Autodesk Inventor part; units mm, degrees
ref_plane "YZ Plane" through (0, 0, 0) normal (1, 0, 0) x (0, 1, 0)
ref_plane "XZ Plane" through (0, 0, 0) normal (0, 1, 0) x (-1, 0, 0)
ref_plane "XY Plane" through (0, 0, 0) normal (0, 0, 1) x (1, 0, 0)
sketch "Sketch1" plane through (0, 0, 0) normal (0, 1, 0) x (-1, 0, 0)
  line L0 (0, 0) -> (0, -2) construction
  line L1 (-2.5, 0) -> (-2.5, -2)
  line L2 (2.5, -2) -> (2.5, 0)
  arc A0 (2.5, 0) -> (-2.5, 0) centre (0, 0) ccw
  arc A1 (-2.5, -2) -> (2.5, -2) centre (0, -2) ccw
  point P0 (0, -1)
  dimension "d0" = 2.5
  dimension "d1" = 2
extrude "Extrusion1" add sketch "Sketch1" along normal blind 2
sketch "Sketch2" plane through (0, 2, 0) normal (0, 1, 0) x (1, 0, 0)
  circle A0 centre (0, 1) radius 1.5
  line L0 (-2.5, 2) -> (-2.5, 0)
  point P0 (0, 0)
  point P1 (-2.5, 1)
  dimension "d4" = 3
extrude "Extrusion2" cut sketch "Sketch2" against normal blind 12.25
fillet "Fillet1" radius 0.5 8 edges at (2.5, 2, -1) (0, 2, -4.5) (-2.5, 2, -1) (0, 2, 2.5) (2.5, 0, -1) (0, 0, -4.5) (-2.5, 0, -1) (0, 0, 2.5)
sketch "Sketch3" plane through (0, 2, 0) normal (0, 1, 0) x (1, 0, 0)
  circle A0 centre (0, 1) radius 1.5
  point P0 (0, 0)
extrude "Extrusion3" add sketch "Sketch3" against normal blind 1.5
properties part number "Ползунок"
Verification items for the finished model (mm, model axes). A direction names the side the tool comes from. Coordinates: 2 decimals unless noted, no trailing zeros. Write each loop counter-clockwise with the first axis right and the second up, starting at its lowest first coordinate (ties: lowest second). Pieces come first, ordered by that corner, then holes. Notation, with made-up numbers: M -37.5,-23 L 7.5,-23 A30 cw 7.5,13 Z; hole C 20.5,-32.5 d8. An arc over 180 degrees is marked long. Use a Markdown table: item, result.
Q1. Set-up check for faces 4 (the face through (-1.11, 0.25, -2.01)), 5 (the face through (2.5, 1, -1)): record each of +Z, -Z, +X, -X, +Y, -Y from which the full face is reachable in a straight line by a thin tool's end or side.
Reply:
| item | result |
|---|---|
| face 4 | -Y |
| face 5 | +Z, -Z, +X, +Y, -Y |
Q2. Sectioned sample at D-D, the plane y = 1.3. Record the boundary of the cut face in (x, z).
Reply:
| item | result |
|---|---|
| outline | M -2.5,-2 A2.5 ccw 2.5,-2 L 2.5,0 A2.5 ccw -2.5,0 Z |
Q3. Thickness scan on line 1 (X direction, y = 0.45, z = -1); line 2 (Z direction, x = 0, y = 0.15); line 3 (Y direction, x = -1, z = 0). Record the ranges inside material, lowest first.
Reply:
| item | result |
|---|---|
| line 1 | x = -2.5 to -1.5, 1.5 to 2.5 |
| line 2 | z = -4.36 to -2.5, 0.5 to 2.36 |
| line 3 | y = 0.5 to 2 |
Q4. Sectioned sample at C-C, the plane x = 0. Record the boundary of the cut face in (y, z).
Reply:
| item | result |
|---|---|
| outline | M 0,-4 A0.5 ccw 0.5,-4.5 L 1.5,-4.5 A0.5 ccw 2,-4 L 2,2 A0.5 ccw 1.5,2.5 L 0.5,2.5 A0.5 ccw 0,2 L 0,0.5 L 0.5,0.5 L 0.5,-2.5 L 0,-2.5 Z |
Q5. Sectioned sample at A-A, the plane z = -1. Record the boundary of the cut face in (x, y), plus the area to 3 significant figures.
Reply:
| item | result |
|---|---|
| outline | M -2.5,0.5 A0.5 ccw -2,0 L -1.5,0 L -1.5,0.5 L 1.5,0.5 L 1.5,0 L 2,0 A0.5 ccw 2.5,0.5 L 2.5,1.5 A0.5 ccw 2,2 L -2,2 A0.5 ccw -2.5,1.5 Z |
| area | 8.29 mm² |
Q6. Draft check along X on faces 1 (the face through (0, 2, -1)), 2 (the face through (0, 0.5, -1)), 3 (the face through (-0.1, 1, -4.5)). Enter one of: +X half, -X half, draft (parallel to the pull), parting line (faces both ways), or undercut.
Reply:
| item | result |
|---|---|
| face 1 | draft |
| face 2 | undercut |
| face 3 | parting line |
Q7. Go/stop test with a flat-tipped pin: P1, Ø1, axis at y = 0.5, z = -3, coming from the -X side. Record where the tip stops, or that it passes through.
Reply:
| item | result |
|---|---|
| P1 | stops at x = -2.45 |
Q8. Sectioned sample at B-B, the plane y = 0.2. Record the boundary of the cut face in (x, z).
Reply:
| item | result |
|---|---|
| outline | M -2.4,-2 A2.4 ccw 2.4,-2 L 2.4,0 A2.4 ccw -2.4,0 Z; hole C 0,-1 d3 |
